```python
from build123d import *

# Parameters (mm, degrees)
SKETCH2_W = 80
SKETCH2_H = 200
SKETCH4_W = 35
SKETCH4_H = 304.864877585


with BuildPart() as part:
    # Sketch2 → Revolve3 (revolve)
    with BuildSketch(Plane.XY, mode=Mode.PRIVATE) as revolve3_sk:
        Polygon((-25, 0), (0, 0), (0, 30), (-80, 30), (-80, 0), align=None)
        Polygon((0, -30), (0, 0), (-25, 0), (-80, 0), (-160, 0), (-160, -30), (-80, -30), align=None)
        with Locations((-40, -130)):
            Rectangle(SKETCH2_W, SKETCH2_H)
    revolve(revolve3_sk.sketch.rotate(Axis((0, -55, 0), (0, 1, 0)), 270), axis=Axis((0, -55, 0), (0, 1, 0)))

    # Sketch4 → Cut-Revolve7 (revolve, cut)
    with BuildSketch(Plane.XY, mode=Mode.PRIVATE) as cut_revolve7_sk:
        with Locations((-17.5, -99.023733968)):
            Rectangle(SKETCH4_W, SKETCH4_H)
    revolve(cut_revolve7_sk.sketch.rotate(Axis((0, -55, 0), (0, 1, 0)), 270), axis=Axis((0, -55, 0), (0, 1, 0)), mode=Mode.SUBTRACT)


solid = part.part
```
Here's how the part is built. I have some questions about the finished solid (model axes, mm). A direction names the side the tool comes from. Give positions to 0.01 mm unless a question says otherwise; leave off trailing zeros. Order: outer loops, then holes, each group sorted by start corner. A loop starts at its lowest first (then second) coordinate and runs counter-clockwise, first axis right, second up. Notation, with made-up numbers: (-25.75, 75) - (-2.75, 75) arc R33 cw to (-2.75, 107) - close; hole circle Ø4 at (-30, -4.75). An arc over 180 degrees is marked (long way). Answer as a JSON object with one key per item and string values. Group by question number.
Item 1: If we section it at C-C on y = -9: Please give me the cut outline in (x, z), and give its area (3 significant figures).
Item 2: If we section it at D-D on z = -49: Please give me the cut outline in (x, y), and give its area (3 significant figures).
Item 3: Which directions (+Z, -Z, +X, -X, +Y, -Y) give clear straight access to the entire face, cutting with the end or side of a thin tool? Please do faces 1 (the flat face through (34, 30, 17)), 2 (the flat face through (33.3, 0, -73.4)), 3 (the flat face through (-73.4, -30, -33.3)).
Item 4: If we section it at A-A on x = 0: Please give me the cut outline in (y, z), and give its area (3 significant figures).
Item 5: If we mould it in two halves opening along X, with no side actions, what happens to faces 4 (the flat face through (17, -230, -34)), 5 (the cylindrical face through (21, -98, 28)), 6 (the cylindrical face through (156.195, -15.21, 34.685))? For each: pulls with the +X half, pulls with the -X half, needs draft (parallel to the pull), parting line crosses it, or undercut.
Item 6: Please list where these lines run through material, in increasing order: probe 1 along X at (y, z) = (-131, 0); probe 2 along Y at (x, z) = (-69, -138.5); probe 3 along X at (y, z) = (-25, 0).
Item 7: For P1, Ø5, axis at y = -145.5, z = -31.5, coming from the +X side; P2, Ø1, axis at x = 89.5, y = -27.5, coming from the -Z side; P3, Ø4, axis at x = 119.5, z = -84.5, coming from the +Y side, each with a flat end and sliding along its axis, tell me the tip position at first contact or that it passes through.
Item 8: If we section it at B-B on z = 0: Please give me the cut outline in (x, y).
Result set:
{
 "1": {"outline": "circle Ø320 at (0, 0); hole circle Ø70 at (0, 0)", "area": "76,600 mm²"},
 "2": {"outline": "(-152.31, -30) - (-63.24, -30) - (-63.24, -230) - (63.24, -230) - (63.24, -30) - (152.31, -30) - (152.31, 0) - (63.24, 0) - (63.24, 30) - (-63.24, 30) - (-63.24, 0) - (-152.31, 0) - close", "area": "38,200 mm²"},
 "3": {"face 1": "+Z, -Z, +X, -X, +Y", "face 2": "+Y", "face 3": "-Y"},
 "4": {"outline": "(-230, -80) - (-30, -80) - (-30, -160) - (0, -160) - (0, -80) - (30, -80) - (30, -35) - (-230, -35) - close; (-230, 35) - (30, 35) - (30, 80) - (0, 80) - (0, 160) - (-30, 160) - (-30, 80) - (-230, 80) - close", "area": "28,200 mm²"},
 "5": {"face 4": "needs draft", "face 5": "undercut", "face 6": "parting line crosses it"},
 "6": {"probe 1": "-80 to -35, 35 to 80", "probe 2": "-30 to 0", "probe 3": "-160 to -35, 35 to 160"},
 "7": {"P1": "x = 74.56", "P2": "z = -132.96", "P3": "y = 0"},
 "8": {"outline": "(-160, -30) - (-80, -30) - (-80, -230) - (-35, -230) - (-35, 30) - (-80, 30) - (-80, 0) - (-160, 0) - close; (35, -230) - (80, -230) - (80, -30) - (160, -30) - (160, 0) - (80, 0) - (80, 30) - (35, 30) - close"}
}
